Autodesk Inventor part; units mm, degrees
ref_plane "YZ Plane" through (0, 0, 0) normal (1, 0, 0) x (0, 1, 0)
ref_plane "XZ Plane" through (0, 0, 0) normal (0, 1, 0) x (-1, 0, 0)
ref_plane "XY Plane" through (0, 0, 0) normal (0, 0, 1) x (1, 0, 0)
sketch "Sketch1" plane through (0, 0, 0) normal (0, 0, 1) x (1, 0, 0)
  circle A0 centre (9.5, 9.5) radius 2.5
  circle A1 centre (40, 40) radius 2.5
  circle A2 centre (40.5, 9.5) radius 2.5
  circle A3 centre (9.5, 40.5) radius 2.5
  line L0 (47.46, 3) -> (27.54, 3)
  line L1 (47.46, 3) -> (47.46, 12.7)
  line L2 (47.46, 12.7) -> (50, 12.7)
  line L3 (50, 12.7) -> (50, 40)
  arc A4 (50, 40) -> (40, 50) centre (40, 40) ccw
  line L4 (10, 50) -> (40, 50)
  arc A5 (10, 50) -> (0, 40) centre (10, 40) ccw
  line L5 (0, 12.7) -> (0, 40)
  line L6 (0, 12.7) -> (2.54, 12.7)
  line L7 (2.54, 12.7) -> (2.54, 3)
  line L8 (22.46, 3) -> (2.54, 3)
  line L9 (22.46, 3) -> (22.46, 12.7)
  line L10 (22.46, 12.7) -> (27.54, 12.7)
  line L11 (27.54, 12.7) -> (27.54, 3)
  circle A6 centre (25, 25) radius 4
  line L12 (25, 25) -> (-22.519, 56.75) construction
  line L13 (-22.519, 56.75) -> (25, 56.75) construction
  line L14 (25, 56.75) -> (25, 25) construction
  line L15 (-28.0183, 56.75) -> (-25.2687, 61.5125)
  line L16 (-25.2687, 61.5125) -> (-19.7694, 61.5125)
  line L17 (-19.7694, 61.5125) -> (-17.0198, 56.75)
  line L18 (-17.0198, 56.75) -> (-19.7694, 51.9875)
  line L19 (-19.7694, 51.9875) -> (-25.2687, 51.9875)
  line L20 (-25.2687, 51.9875) -> (-28.0183, 56.75)
  line L21 (-19.7694, 61.5125) -> (-25.2687, 51.9875) construction
  circle A7 centre (-22.519, 56.75) radius 6.985
  circle A8 centre (40, 40) radius 5.04
  circle A9 centre (40.5, 9.5) radius 5.04
  circle A10 centre (9.5, 9.5) radius 5.04
  arc A11 (35.8521, 7.5509) -> (14.1479, 7.5509) centre (25, 3) ccw
  arc A12 (4.6471, 8.1396) -> (-26.3996, 50.9421) centre (-68.7442, -12.4335) ccw
  arc A13 (-18.6385, 62.5579) -> (39.9595, 45.0398) centre (39.1237, 149.0084) ccw
  circle A14 centre (25, 25) radius 6.54
  line L22 (-26.3996, 50.9421) -> (-15.682, 43.7811) construction
  line L23 (-18.6385, 62.5579) -> (-6.4516, 54.4152) construction
  line L24 (45.54, 9.5) -> (45.04, 40)
  circle A15 centre (40, 40) radius 1.75
  circle A16 centre (40.5, 9.5) radius 1.75
  circle A17 centre (9.5, 9.5) radius 1.75
  circle A18 centre (9.5, 40.5) radius 3.2571
  point P0 (0, 0)
  dimension "d0" = 57.15
  dimension "d1" = 31.75
  dimension "d3" = 120
  dimension "d4" = 120
  dimension "d5" = 9.525
  dimension "d6" = 13.97
  dimension "d7" = 2.54
  dimension "d8" = 2.54
  dimension "d9" = 2.54
  dimension "d11" = 2.54
extrude "Extrusion1" add sketch "Sketch1" along normal blind 8.175 contours A0 | A1 | A2 | A9 | A13 A8 L24 A9 A11 A10 A12 L5 A5 | A5 L5 A12 A7 A13 | A7 | A8 | A10 | L15 L16 L17 L18 L19 L20
sketch "Sketch2" plane through (0, 0, 8.175) normal (0, 0, 1) x (1, 0, 0)
  line L0 (-25.2687, 51.9875) -> (-28.0183, 56.75)
  line L1 (-28.0183, 56.75) -> (-25.2687, 61.5125)
  line L2 (-25.2687, 61.5125) -> (-19.7694, 61.5125)
  line L3 (-19.7694, 61.5125) -> (-17.0198, 56.75)
  line L4 (-17.0198, 56.75) -> (-19.7694, 51.9875)
  line L5 (-19.7694, 51.9875) -> (-25.2687, 51.9875)
  point P0 (0, 0)
extrude "Extrusion2" add sketch "Sketch2" along normal blind 15.875
chamfer "Chamfer1" distance 1 angle 45 6 edges at (-22.519, 61.5125, 24.05) (-26.6435, 59.1312, 24.05) (-26.6435, 54.3687, 24.05) (-22.519, 51.9875, 24.05) (-18.3946, 59.1312, 24.05) (-18.3946, 54.3687, 24.05)
properties part number "ArmGearMount"
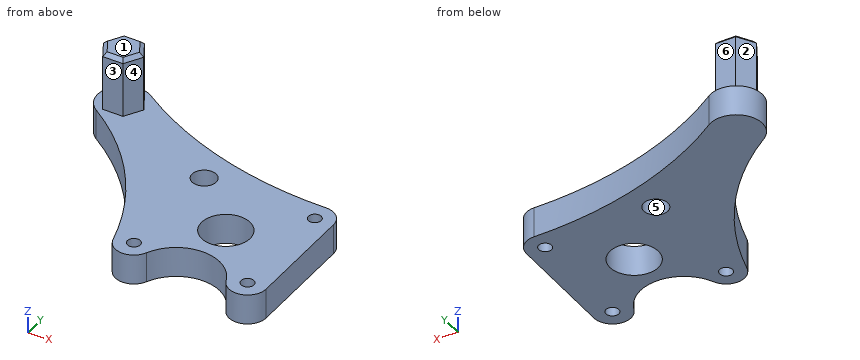
Work out the finished part from the listing and answer in its coordinate system (mm). Face numbers are marked on the shaded views. A direction names the side the tool comes from. Give positions to 0.01 mm unless a question says otherwise; leave off trailing zeros. Loops run counter-clockwise (first coordinate to the right, second up) from the corner with the lowest first, then second, coordinate; pieces in that order, holes last. Notation, with made-up numbers: (89.25, -27) - (93.25, -27) arc R19 ccw to (93.25, -15) - close; hole circle Ø5 at (-12, 0.5). An arc over 180 degrees is marked (long way). Answer in a Markdown table with one row per item.
(1) For a pull along X with two mould halves and no side action, classify the marked faces 4, 5 and 6 as pulls with the +X half, pulls with the -X half, needs draft (parallel to the pull), parting line crosses it, or undercut.
Results list:
| item | result |
|---|---|
| face 4 | pulls with the +X half |
| face 5 | undercut |
| face 6 | needs draft |
(2) Section B-B (y = 29) is taken. Give the vertices of the cut face in (x, z) (3 decimals).
Results list:
| item | result |
|---|---|
| outline | (-4.769, 0) - (19.826, 0) - (19.826, 8.175) - (-4.769, 8.175) - close; (30.174, 0) - (45.22, 0) - (45.22, 8.175) - (30.174, 8.175) - close |
(3) Section C-C (x = 9.5) is taken. Give the vertices of the cut face in (y, z) (3 decimals), and give its area (3 significant figures).
Results list:
| item | result |
|---|---|
| outline | (4.46, 0) - (7.75, 0) - (7.75, 8.175) - (4.46, 8.175) - close; (11.25, 0) - (37.243, 0) - (37.243, 8.175) - (11.25, 8.175) - close; (43.757, 0) - (49.346, 0) - (49.346, 8.175) - (43.757, 8.175) - close |
| area | 285 mm² |
(4) Section D-D (z = 16.5) is taken. Give the vertices of the cut face in (x, y), and give its area (3 significant figures).
Results list:
| item | result |
|---|---|
| outline | (-28.02, 56.75) - (-25.27, 51.99) - (-19.77, 51.99) - (-17.02, 56.75) - (-19.77, 61.51) - (-25.27, 61.51) - close |
| area | 78.6 mm² |
(5) A tool of negligible diameter and unlimited length cuts with its end or side. For the marked faces 1, 2 and 3, from which of +Z, -Z, +X, -X, +Y, -Y can it reach the whole face along a straight path? Write none if from no direction.
Results list:
| item | result |
|---|---|
| face 1 | +Z, +X, -X, +Y, -Y |
| face 2 | +Z, -X, +Y |
| face 3 | +Z, +X, -X, -Y |
(6) Flat-ended cylindrical pins translate along their axes: pin 1 Ø17 at (x, y) = (25, 25) entering from +Z (3 decimals); pin 2 Ø6 at (x, z) = (-21.5, 16) entering from -Y; pin 3 Ø6 at (x, z) = (30.5, 3.5) entering from +Y. Find the tip coordinate at first contact, or state that the pin passes through.
Results list:
| item | result |
|---|---|
| pin 1 | stops at z = 8.175 |
| pin 2 | stops at y = 51.99 |
| pin 3 | stops at y = 45.69 |
(7) Consider L1, parallel to Y at x = 40, z = 5.75; L2, parallel to Y at x = 9.5, z = 1.5; L3, parallel to Z at x = 39, y = 24 (3 decimals). Determine where each line is inside the solid, lowest interval first. Write a range as [from, to].
Results list:
| item | result |
|---|---|
| L1 | y = [4.48, 7.82], [11.18, 38.25], [41.75, 45.04] |
| L2 | y = [4.46, 7.75], [11.25, 37.24], [43.76, 49.35] |
| L3 | z = [0, 8.175] |
(8) Section A-A (x = 25) is taken. Give the vertices of the cut face in (y, z) (3 decimals), and give its area (3 significant figures).
Results list:
| item | result |
|---|---|
| outline | (14.768, 0) - (18.46, 0) - (18.46, 8.175) - (14.768, 8.175) - close; (31.54, 0) - (46, 0) - (46, 8.175) - (31.54, 8.175) - close |
| area | 148 mm² |
